Can you work these out from the model? Positions are in its coordinate system, mm. Face numbers are marked on the shaded views. A direction names the side the tool comes from. Round coordinates to 2 decimals unless told otherwise and drop trailing zeros. Order: outer loops, then holes, each group sorted by start corner. A loop starts at its lowest first (then second) coordinate and runs counter-clockwise, first axis right, second up.
Q1. If we section it at D-D (z = -38): Please give me the cut outline in (x, y) (1 decimal).
Q2. Will these pins go through, and if not, where does the flat tip stop? P1, Ø6.5, axis at y = 8.5, z = -36.5, coming from the -X side (3 decimals); P2, Ø6.5, axis at y = 8.5, z = -46.5, coming from the +X side (3 decimals); P3, Ø4, axis at x = -3.5, z = -54, coming from the -Y side; P4, Ø4.5, axis at x = -9.525, z = -69.85, coming from the +Y side.
Q3. If we section it at C-C (x = 0): Count the separate pieces of the cut face and the enclosed holes in it, plus the area to 3 significant figures.
Q4. For the marked faces 1, 2, 3, 4 and 5, which set-ups out of +Z, -Z, +X, -X, +Y, -Y let a thin tool reach every point of the face, with its end or its side?
Q5. If we section it at A-A (z = -69.85): Please give me the cut outline in (x, y) (1 decimal).
Q6. If I drill on line 1 (X direction, y = 5.25, z = -69.85) (3 decimals); line 2 (Y direction, x = 15, z = -30); line 3 (Y direction, x = 6.5, z = 3), over which ranges is the centre line in solid material (lowest first)?
from build123d import *

# Parameters (mm, degrees)
BOSS_EXTRUDE1_DEPTH         = 13.352390271
SKETCH4_R                   = 28.575
BOSS_EXTRUDE2_DEPTH         = 19.05
SKETCH5_R                   = 31.75
SKETCH5_R_2                 = 28.575
BOSS_EXTRUDE3_DEPTH         = 3.175
F_3_8_16_TAPPED_HOLE1_D     = 7.9375
F_1_4_20_TAPPED_HOLE2_D     = 5.1054
F_1_4_20_TAPPED_HOLE2_DEPTH = 118.27002
F_1_4_20_TAPPED_HOLE2_TIP   = 1.533816902
SKETCH2_R                   = 6.35
BOSS_EXTRUDE6_DEPTH         = 37.990390271
SKETCH23_W                  = 0.4064
SKETCH23_H                  = 0.9906


with BuildPart() as part:
    # Sketch1 → Boss-Extrude1 (new body)
    with BuildSketch(Plane(origin=(0, 0, 0), x_dir=(1, 0, 0), z_dir=(0, 1, 0))):
        with BuildLine():
            Line((-15.875, 0), (-15.875, 79.375))
            Line((-15.875, 79.375), (15.875, 79.375))
            Line((15.875, 79.375), (15.875, 0))
            ThreePointArc((15.875, 0), (0, -15.875), (-15.875, 0))
        make_face()
    extrude(amount=BOSS_EXTRUDE1_DEPTH)

    # Sketch4 → Boss-Extrude2 (add)
    with BuildSketch(Plane.XZ):
        Circle(SKETCH4_R)
    extrude(amount=BOSS_EXTRUDE2_DEPTH)

    # Sketch5 → Boss-Extrude3 (add)
    with BuildSketch(Plane.XZ):
        with Locations(Location((0, 0, 0), (0, 0, 240))):
            Circle(SKETCH5_R)
        Circle(SKETCH5_R_2, mode=Mode.SUBTRACT)
    extrude(amount=BOSS_EXTRUDE3_DEPTH)

    # 3/8-16 Tapped Hole1 (through all)
    with Locations(Plane(origin=(0, 0, -79.375), x_dir=(-1, 0, 0), z_dir=(0, 0, -1))):
        with Locations((0, 6.676195135)):
            Hole(F_3_8_16_TAPPED_HOLE1_D / 2)

    # 1/4-20 Tapped Hole2
    with Locations(Plane(origin=(0, 13.352390271, 0), x_dir=(1, 0, 0), z_dir=(0, 1, 0))):
        with Locations((-9.525, 69.85), (9.525, 69.85), (0, 11.1125)):
            Hole(F_1_4_20_TAPPED_HOLE2_D / 2, depth=F_1_4_20_TAPPED_HOLE2_DEPTH)
            with Locations((0, 0, -(F_1_4_20_TAPPED_HOLE2_DEPTH + F_1_4_20_TAPPED_HOLE2_TIP / 2))):  # 118° drill point
                Cone(0, F_1_4_20_TAPPED_HOLE2_D / 2, F_1_4_20_TAPPED_HOLE2_TIP, mode=Mode.SUBTRACT)

    # Sketch22 → Cut-Revolve2 (revolve, cut)
    with BuildSketch(Plane.XY, mode=Mode.PRIVATE) as cut_revolve2_sk:
        Polygon((28.575, -8.5725), (26.035, -11.1125), (28.575, -13.6525), align=None)
    revolve(cut_revolve2_sk.sketch.rotate(Axis((0, -19.050000001, 0), (0, 1, 0)), 90), axis=Axis((0, -19.050000001, 0), (0, 1, 0)), mode=Mode.SUBTRACT)

    # Sketch2 → Boss-Extrude6 (add)
    with BuildSketch(Plane(origin=(0, 13.352390271, 0), x_dir=(1, 0, 0), z_dir=(0, 1, 0))):
        Circle(SKETCH2_R)
    extrude(amount=-BOSS_EXTRUDE6_DEPTH)

    # Sketch23 → Cut-Revolve4 (revolve, cut)
    with BuildSketch(Plane(origin=(0, 0, 0), x_dir=(0, 0, -1), z_dir=(1, 0, 0)), mode=Mode.PRIVATE) as cut_revolve4_sk:
        with Locations((-6.1468, -16.384583292)):
            Rectangle(SKETCH23_W, SKETCH23_H)
    revolve(cut_revolve4_sk.sketch.rotate(Axis((0, -24.638, 0), (0, 1, 0)), 180), axis=Axis((0, -24.638, 0), (0, 1, 0)), mode=Mode.SUBTRACT)


solid = part.part
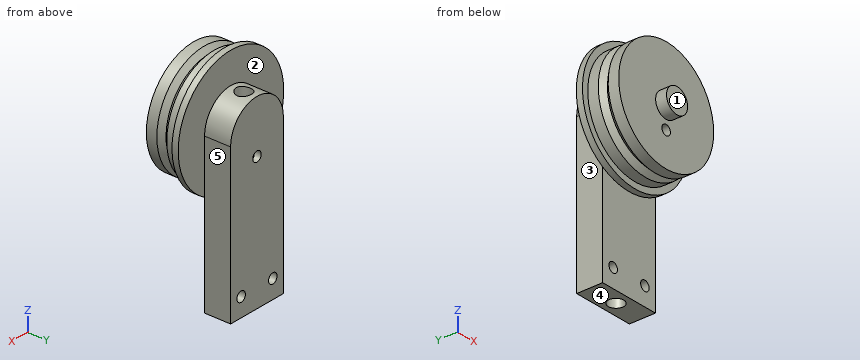
Solution:
1. outline: (-15.9, 0) - (15.9, 0) - (15.9, 13.4) - (-15.9, 13.4) - close; hole circle Ø7.9 at (0, 6.7)
2. P1: stops at x = -15.875
2. P2: stops at x = 15.875
2. P3: stops at y = 0
2. P4: passes through
3. separate pieces: 3
3. enclosed holes: 2
3. area: 1,660 mm2
4. face 1: +Z, -Z, +X, -X, -Y
4. face 2: +Z, +Y
4. face 3: +Z, -Z, -X, +Y
4. face 4: -Z, +X, -X, +Y, -Y
4. face 5: +Z, -Z, +X, +Y
5. outline: (-15.9, 0) - (-12.1, 0) - (-12.1, 13.4) - (-15.9, 13.4) - close; (-7, 0) - (7, 0) - (7, 13.4) - (-7, 13.4) - close; (12.1, 0) - (15.9, 0) - (15.9, 13.4) - (12.1, 13.4) - close; hole circle Ø7.9 at (0, 6.7)
6. line 1: x = -15.875 to -12.078, -6.972 to -3.704, 3.704 to 6.972, 12.078 to 15.875
6. line 2: y = 0 to 13.35
6. line 3: y = -19.05 to 13.35
